Check sheet for the modelled part. Datum: model origin and axes. Units: mm. Round coordinates to 2 decimals unless told otherwise and drop trailing zeros. Write each loop counter-clockwise with the first axis right and the second up, starting at its lowest first coordinate (ties: lowest second). Pieces come first, ordered by that corner, then holes. Notation, with made-up numbers: (-36.75, -35) -> (-12.75, -35) arc R27 ccw to (-12.75, 2) -> close; hole circle Ø8 at (46.25, 21.25). An arc over 180 degrees is marked (long way). One line per item, written item: value.
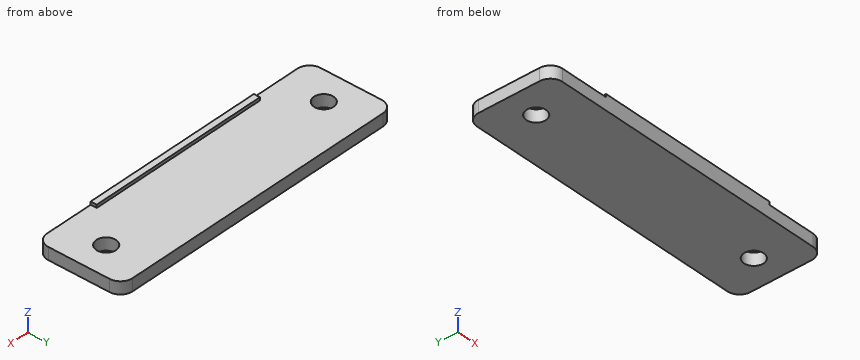
from build123d import *

# Parameters (mm, degrees)
SKETCH2_W           = 50
SKETCH2_H           = 14
BOSS_EXTRUDE1_DEPTH = 2.5
SKETCH4_OUTSIDE_W   = 62.396
SKETCH4_OUTSIDE_H   = 26.396
SKETCH4_OUTSIDE_W_2 = 30
SKETCH4_OUTSIDE_H_2 = 1
CUT_EXTRUDE1_DEPTH  = 0.5
SKETCH5_R           = 1.6
CUT_EXTRUDE2_DEPTH  = 2
FILLET2_R           = 2


with BuildPart() as part:
    # Sketch2 → Boss-Extrude1 (new body)
    with BuildSketch(Plane.XY):
        Rectangle(SKETCH2_W, SKETCH2_H)
    extrude(amount=BOSS_EXTRUDE1_DEPTH)

    # Sketch4 outside → Cut-Extrude1 (cut)
    with BuildSketch(Plane.XY.offset(2.5)):
        Rectangle(SKETCH4_OUTSIDE_W, SKETCH4_OUTSIDE_H)
        with Locations((0, -6.5)):
            Rectangle(SKETCH4_OUTSIDE_W_2, SKETCH4_OUTSIDE_H_2, mode=Mode.SUBTRACT)
    extrude(amount=-CUT_EXTRUDE1_DEPTH, mode=Mode.SUBTRACT)

    # Sketch5 → Cut-Extrude2 (cut)
    with BuildSketch(Plane.XY.offset(2)):
        with Locations((-20, 0)):
            Circle(SKETCH5_R)
        with Locations((20, 0)):
            Circle(SKETCH5_R)
    extrude(amount=-CUT_EXTRUDE2_DEPTH, mode=Mode.SUBTRACT)

    # Fillet2
    fillet2_edges = [part.edges().sort_by_distance(p)[0] for p in [
        (25, -7, 1),
        (-25, -7, 1),
        (-25, 7, 1),
        (25, 7, 1),
    ]]
    fillet(fillet2_edges, radius=FILLET2_R)


solid = part.part
Item 1: Material ranges on line 1 along X through (y, z) = (-1, 1.2); line 2 along X through (y, z) = (-0.5, 0.55); line 3 along Y through (x, z) = (20, 0.75), recorded low to high.
Result set:
line 1: -25 to -21.25, -18.75 to 18.75, 21.25 to 25
line 2: -25 to -21.52, -18.48 to 18.48, 21.52 to 25
line 3: -7 to -1.6, 1.6 to 7
Item 2: Sectioned sample at C-C (x = -20). Enter the section's corners in (y, z).
Result set:
outline: (-7, 0) -> (-1.6, 0) -> (-1.6, 2) -> (-7, 2) -> close; (1.6, 0) -> (7, 0) -> (7, 2) -> (1.6, 2) -> close
Item 3: Sectioned sample at D-D (x = 14). Enter the section's corners in (y, z), then the cut area to 3 significant figures.
Result set:
outline: (-7, 0) -> (7, 0) -> (7, 2) -> (-6, 2) -> (-6, 2.5) -> (-7, 2.5) -> close
area: 28.5 mm^2
Item 4: Sectioned sample at A-A (z = 1.5). Enter the section's corners in (x, y).
Result set:
outline: (-25, -5) arc R2 ccw to (-23, -7) -> (23, -7) arc R2 ccw to (25, -5) -> (25, 5) arc R2 ccw to (23, 7) -> (-23, 7) arc R2 ccw to (-25, 5) -> close; hole circle Ø3.2 at (-20, 0); hole circle Ø3.2 at (20, 0)
Item 5: Sectioned sample at B-B (y = 0). Enter the section's corners in (x, z).
Result set:
outline: (-25, 0) -> (-21.6, 0) -> (-21.6, 2) -> (-25, 2) -> close; (-18.4, 0) -> (18.4, 0) -> (18.4, 2) -> (-18.4, 2) -> close; (21.6, 0) -> (25, 0) -> (25, 2) -> (21.6, 2) -> close
Item 6: Depth check by flat-ended pin: pin 1 (5 mm diameter, centred on x = 4.5, y = 1.5, fed in from +Z); pin 2 (0.6 mm diameter, centred on y = -6.5, z = 2, fed in from -X); pin 3 (0.6 mm diameter, centred on x = -1, z = 2.5, fed in from +Y); pin 4 (1.9 mm diameter, centred on x = 20, y = 0, fed in from -Z). Enter the tip coordinate at first touch or a pass-through.
Result set:
pin 1: z = 2
pin 2: x = -24.6
pin 3: y = -6
pin 4: through
